Here's how the part is built. I have some questions about the finished solid (model axes, mm). A direction names the side the tool comes from. Round coordinates to 2 decimals unless told otherwise and drop trailing zeros. Answer as CSV lines item,"result".
```python
from build123d import *

# Parameters (mm, degrees)
SKETCH1_W           = 30
SKETCH1_H           = 60
BOSS_EXTRUDE1_DEPTH = 250
SKETCH3_R           = 4.5
SKETCH3_R_2         = 1.8
CUT_EXTRUDE1_DEPTH  = 258.536405194
SKETCH4_R           = 5.1
CUT_EXTRUDE2_DEPTH  = 10


with BuildPart() as part:
    # Sketch1 → Boss-Extrude1 (new, symmetric)
    with BuildSketch(Plane.XY):
        Rectangle(SKETCH1_W, SKETCH1_H)
    extrude(amount=BOSS_EXTRUDE1_DEPTH, both=True)

    # Sketch3 → Cut-Extrude1 (cut, through all)
    with BuildSketch(Plane.XZ.offset(30)):
        with Locations(Location((3, 0, 0), (0, 0, 270))):
            Circle(SKETCH3_R)
        with Locations(Location((11, 0, 0), (0, 0, 270))):
            Circle(SKETCH3_R_2)
        with Locations(Location((3, -8, 0), (0, 0, 270))):
            Circle(SKETCH3_R_2)
        with Locations(Location((-5, 0, 0), (0, 0, 270))):
            Circle(SKETCH3_R_2)
        with Locations(Location((3, 8, 0), (0, 0, 270))):
            Circle(SKETCH3_R_2)
    extrude(amount=-CUT_EXTRUDE1_DEPTH, mode=Mode.SUBTRACT)

    # Sketch4 → Cut-Extrude2 (cut)
    with BuildSketch(Plane.XZ.offset(30)):
        with Locations(Location((3, 0, 0), (0, 0, 270))):
            Circle(SKETCH4_R)
    cut_extrude2 = extrude(amount=-CUT_EXTRUDE2_DEPTH, mode=Mode.SUBTRACT)

    # Mirror1: Cut-Extrude2 across plane
    add(cut_extrude2.mirror(Plane.ZX), mode=Mode.SUBTRACT)


solid = part.part
```
1. On a 3-axis mill with a long thin cutter (end or side, diameter ignored), from which of +Z, -Z, +X, -X, +Y, -Y can I reach the whole of each face in a straight line? I mean faces 1 (the face through (4.532, -25.07, -4.864)), 2 (the face through (0, 0, 250)), 3 (the face through (4.532, 25.07, -4.864)). Say none if no direction works.
Numbers:
face 1,"-Y"
face 2,"+Z, +X, -X, +Y, -Y"
face 3,"+Y"
2. If we mould it in two halves opening along Z, with no side actions, what happens to faces 4 (the face through (0.3, -0.3, 3.6)), 5 (the face through (-4, -30, 4)), 6 (the face through (0, 0, -250))? For each: released by +Z, released by -Z, zero draft, split by the parting line, or undercut.
Numbers:
face 4,"undercut"
face 5,"zero draft"
face 6,"released by -Z"
3. If I drill on line 1 (X direction, y = 26.25, z = 0); line 2 (X direction, y = 9, z = 0); line 3 (X direction, y = 6.5, z = 8), over which ranges is the centre line in solid material (lowest first)?
Numbers:
line 1,"x = -15 to -6.8, -3.2 to -2.1, 8.1 to 9.2, 12.8 to 15"
line 2,"x = -15 to -6.8, -3.2 to -1.5, 7.5 to 9.2, 12.8 to 15"
line 3,"x = -15 to 1.2, 4.8 to 15"
4. For pin 1 Ø3 at (x, z) = (0.5, -2) entering from -Y; pin 2 Ø4 at (x, z) = (-5, 0) entering from +Y, each with a flat end and sliding along its axis, tell me the tip position at first contact or that it passes through.
Numbers:
pin 1,"stops at y = -20"
pin 2,"stops at y = 30"
